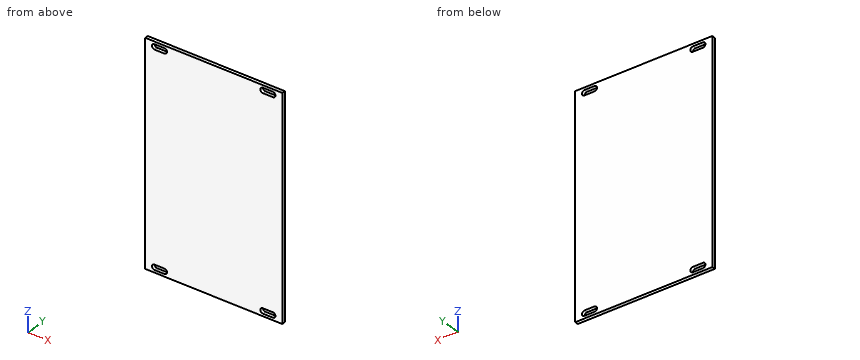
from build123d import *

# Parameters (mm, degrees)
F0_W     = 80.9
F0_H     = 128.5
F1_DEPTH = 2


with BuildPart() as f1:
    # F0 (on Front) → F1 (new body)
    with BuildSketch(Plane.XZ):
        Rectangle(F0_W, F0_H)
        with BuildLine():
            ThreePointArc((-34.95, -62.8), (-36.45, -61.3), (-34.95, -59.8))
            Line((-34.95, -59.8), (-29.05, -59.8))
            ThreePointArc((-29.05, -59.8), (-27.55, -61.3), (-29.05, -62.8))
            Line((-29.05, -62.8), (-34.95, -62.8))
        make_face(mode=Mode.SUBTRACT)
        with BuildLine():
            ThreePointArc((29.05, -62.8), (27.55, -61.3), (29.05, -59.8))
            Line((29.05, -59.8), (34.95, -59.8))
            ThreePointArc((34.95, -59.8), (36.45, -61.3), (34.95, -62.8))
            Line((34.95, -62.8), (29.05, -62.8))
        make_face(mode=Mode.SUBTRACT)
        with BuildLine():
            ThreePointArc((-34.95, 59.8), (-36.45, 61.3), (-34.95, 62.8))
            Line((-34.95, 62.8), (-29.05, 62.8))
            ThreePointArc((-29.05, 62.8), (-27.55, 61.3), (-29.05, 59.8))
            Line((-29.05, 59.8), (-34.95, 59.8))
        make_face(mode=Mode.SUBTRACT)
        with BuildLine():
            ThreePointArc((29.05, 59.8), (27.55, 61.3), (29.05, 62.8))
            Line((29.05, 62.8), (34.95, 62.8))
            ThreePointArc((34.95, 62.8), (36.45, 61.3), (34.95, 59.8))
            Line((34.95, 59.8), (29.05, 59.8))
        make_face(mode=Mode.SUBTRACT)
    extrude(amount=F1_DEPTH)


solid = f1.part
Verification items for the finished model (mm, model axes). Coordinates: 2 decimals unless noted, no trailing zeros. Order: outer loops, then holes, each group sorted by start corner. A loop starts at its lowest first (then second) coordinate and runs counter-clockwise, first axis right, second up. Notation, with made-up numbers: M 39,89.25 L 70,89.25 A13 ccw 70,99.25 Z; hole C -30.5,-30.5 d2. An arc over 180 degrees is marked long. Return JSON: item names as keys, results as strings.
1) Gauge pin test, flat end, axial feed: pin 1 (2 mm diameter, centred on x = 22.5, z = -32.5, fed in from +Y). Record the tip position at first contact, or that the pin passes through.
Answer list:
{"pin 1": "y = 0"}
2) Thickness scan on L1, parallel to Z at x = -33.5, y = -0.6. Record the ranges inside material, lowest first. Write a range as [from, to].
Answer list:
{"L1": "[-64.25, -62.8], [-59.8, 59.8], [62.8, 64.25]"}
3) Cross-section at B-B, the plane x = 31. Record the boundary of the cut face in (y, z), and give its area (3 significant figures).
Answer list:
{"outline": "M -2,-64.25 L 0,-64.25 L 0,-62.8 L -2,-62.8 Z; M -2,-59.8 L 0,-59.8 L 0,59.8 L -2,59.8 Z; M -2,62.8 L 0,62.8 L 0,64.25 L -2,64.25 Z", "area": "245 mm2"}
4) Cross-section at A-A, the plane z = 61.3. Record the boundary of the cut face in (x, y).
Answer list:
{"outline": "M -40.45,-2 L -36.45,-2 L -36.45,0 L -40.45,0 Z; M -27.55,-2 L 27.55,-2 L 27.55,0 L -27.55,0 Z; M 36.45,-2 L 40.45,-2 L 40.45,0 L 36.45,0 Z"}
